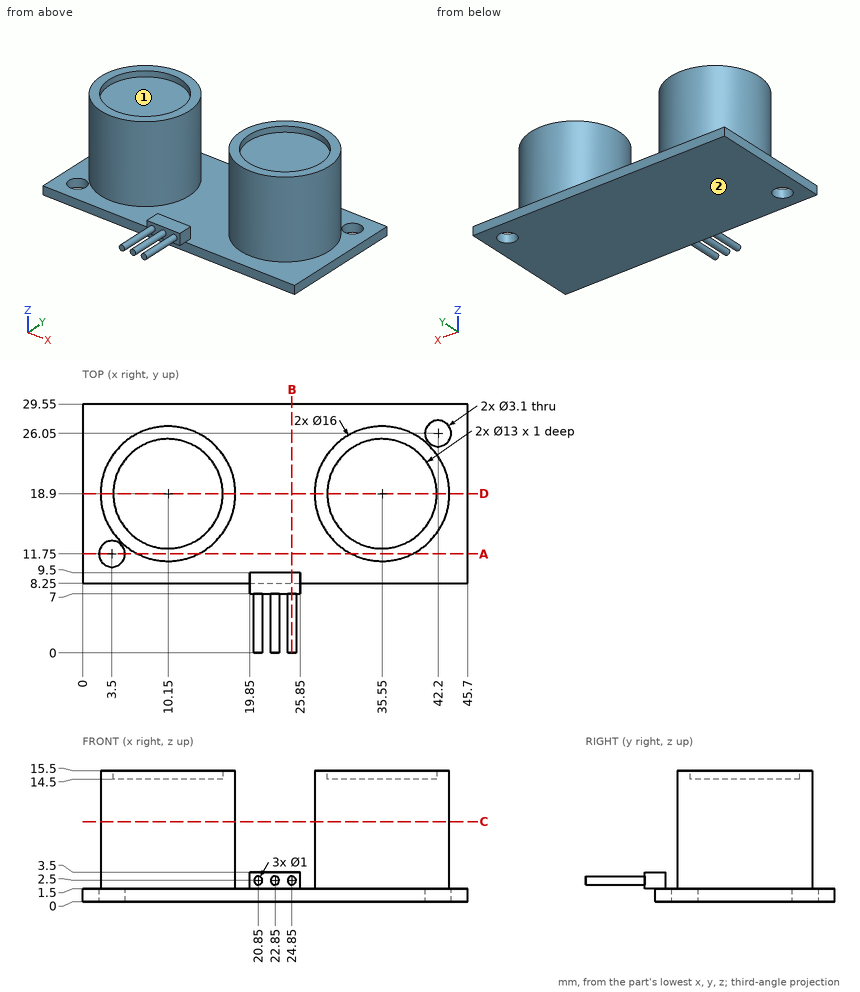
Study the drawing (mm; zero at the part's minimum x, y, z) and answer. Give positions to 0.01 mm unless a question says otherwise; leave off trailing zeros. Loops run counter-clockwise (first coordinate to the right, second up) from the corner with the lowest first, then second, coordinate; pieces in that order, holes last. Notation, with made-up numbers: M 81,9.5 L 110,9.5 A22 ccw 110,43.5 Z; hole C -20.5,32.5 d5. An arc over 180 degrees is marked long. One line per item, written item: value. Start each with the question number.
1. Find section D-D (y = 18.9). Give the vertices of the cut face in (x, z), and give its area (3 significant figures).
2. Find section A-A (y = 11.75). Give the vertices of the cut face in (x, z).
3. Find section B-B (x = 24.85). Give the vertices of the cut face in (y, z).
4. Find section C-C (z = 9.5). Give the vertices of the cut face in (x, y), and give its area (3 significant figures).
5. Find the intervals of material crossed by probe 1 along Y at (x, z) = (42.2, 1); probe 2 along Y at (x, z) = (35.55, 14.95); probe 3 along Z at (x, y) = (11, 14.25), in increasing order.
6. Determine the mould class of the marked faces 1 and 2 for opening direction X: released by +X, released by -X, zero draft, split by the parting line, or undercut.
7. Each of these flat-tipped pins is pushed along its axis until it touches: P1, Ø5, axis at y = 20.5, z = 6, coming from the -X side; P2, Ø6.5, axis at x = 36.5, y = 15.5, coming from the +Z side; P3, Ø1, axis at x = 35.5, z = 6.5, coming from the +Y side; P4, Ø2.5, axis at x = 42.2, y = 26.05, coming from the -Z side. Where does it stop, or does it pass through?
Reported:
1. outline: M 0,0 L 45.7,0 L 45.7,1.5 L 43.55,1.5 L 43.55,15.5 L 42.05,15.5 L 42.05,14.5 L 29.05,14.5 L 29.05,15.5 L 27.55,15.5 L 27.55,1.5 L 18.15,1.5 L 18.15,15.5 L 16.65,15.5 L 16.65,14.5 L 3.65,14.5 L 3.65,15.5 L 2.15,15.5 L 2.15,1.5 L 0,1.5 Z
1. area: 491 mm²
2. outline: M 0,0 L 1.95,0 L 1.95,1.5 L 0,1.5 Z; M 5.05,0 L 45.7,0 L 45.7,1.5 L 39.14,1.5 L 39.14,15.5 L 31.96,15.5 L 31.96,1.5 L 13.74,1.5 L 13.74,15.5 L 6.56,15.5 L 6.56,1.5 L 5.05,1.5 Z
3. outline: M 0,2 L 7,2 L 7,1.5 L 8.25,1.5 L 8.25,0 L 29.55,0 L 29.55,1.5 L 9.5,1.5 L 9.5,3.5 L 7,3.5 L 7,3 L 0,3 Z
4. outline: C 10.15,18.9 d16; C 35.55,18.9 d16
4. area: 402 mm²
5. probe 1: y = 8.25 to 24.5, 27.6 to 29.55
5. probe 2: y = 10.9 to 12.4, 25.4 to 26.9
5. probe 3: z = 0 to 14.5
6. face 1: undercut
6. face 2: zero draft
7. P1: stops at x = 2.15
7. P2: stops at z = 15.5
7. P3: stops at y = 26.9
7. P4: passes through
